Model file for the job. Use its own axes, mm. A direction names the side the tool comes from. Coordinates: 2 decimals unless noted, no trailing zeros. Order: outer loops, then holes, each group sorted by start corner. A loop starts at its lowest first (then second) coordinate and runs counter-clockwise, first axis right, second up.
from build123d import *

# Parameters (mm, degrees)
EXTRUDE_1_DEPTH     = 2.5
SKETCH_2_R          = 1.4
CUT_EXTRUDE_1_DEPTH = 0.1


with BuildPart() as part:
    # 草图1 → 凸台-拉伸1 (new body, symmetric)
    with BuildSketch(Plane(origin=(0, 0, 0), x_dir=(0, 0, -1), z_dir=(1, 0, 0))):
        with BuildLine():
            Line((6.4, 80), (18.6, 80))
            Line((18.6, 80), (18.6, 71.8744))
            ThreePointArc((18.6, 71.8744), (17.1, 70.3744), (18.6, 68.8744))
            Line((18.6, 68.8744), (21.4, 68.8744))
            ThreePointArc((21.4, 68.8744), (22.9, 70.3744), (21.4, 71.8744))
            Line((21.4, 71.8744), (21.4, 80))
            Line((21.4, 80), (25, 80))
            Line((25, 80), (25, 0))
            Line((25, 0), (0, 0))
            Line((0, 0), (0, 80))
            Line((0, 80), (3.6, 80))
            Line((3.6, 80), (3.6, 71.8744))
            ThreePointArc((3.6, 71.8744), (2.1, 70.3744), (3.6, 68.8744))
            Line((3.6, 68.8744), (6.4, 68.8744))
            ThreePointArc((6.4, 68.8744), (7.9, 70.3744), (6.4, 71.8744))
            Line((6.4, 71.8744), (6.4, 80))
        make_face()
    extrude(amount=EXTRUDE_1_DEPTH, both=True)

    # 草图2 → 切除-拉伸1 (cut)
    with BuildSketch(Plane(origin=(0, 68.8744, 0), x_dir=(1, 0, 0), z_dir=(0, 1, 0))):
        with Locations((0, 20)):
            Circle(SKETCH_2_R)
        with Locations((0, 5)):
            Circle(SKETCH_2_R)
    extrude(amount=-CUT_EXTRUDE_1_DEPTH, mode=Mode.SUBTRACT)


solid = part.part
Q1. Probe line 1 (Y direction, x = 0.4, z = -3.5); line 2 (Y direction, x = -0.9, z = -17.25); line 3 (Y direction, x = -0.2, z = -4.5). List the from-to ranges inside material, lowest first.
Established:
line 1: y = 0 to 68.88, 71.87 to 80
line 2: y = 0 to 69.72, 71.03 to 80
line 3: y = 0 to 68.77
Q2. Which spindle directions (+Z, -Z, +X, -X, +Y, -Y) get a long thin tool onto all of the face, cutting with end or side? Do faces 5 (the face through (0, 80, -2)), 6 (the face through (2, 68.874, -5)), 7 (the face through (0, 70.4, -17.1)). Say none if no direction does.
Established:
face 5: +Z, -Z, +X, -X, +Y
face 6: +X, -X, +Y
face 7: +X, -X
Q3. Drop a flat-ended pin along its axis: P1, Ø2, axis at x = 1.5, z = -5, coming from the +Y side. Give the stop position or say it passes through.
Established:
P1: stops at y = 68.87
Q4. Cut at A-A, the plane z = -5. List the corners of the cut face in (x, y).
Established:
outline: (-2.5, 0) - (2.5, 0) - (2.5, 68.87) - (1.4, 68.87) - (1.4, 68.77) - (-1.4, 68.77) - (-1.4, 68.87) - (-2.5, 68.87) - close
Q5. Mould opens along Y. For faces 1 (the face through (0, 0, -13)), 2 (the face through (-2, 68.874, -20)), 3 (the face through (0, 70.3, -7.9)), 4 (the face through (0, 70.4, -2.1)) say: pulls with the +Y half, pulls with the -Y half, needs draft (parallel to the pull), parting line crosses it, or undercut.
Established:
face 1: pulls with the -Y half
face 2: pulls with the +Y half
face 3: undercut
face 4: undercut
